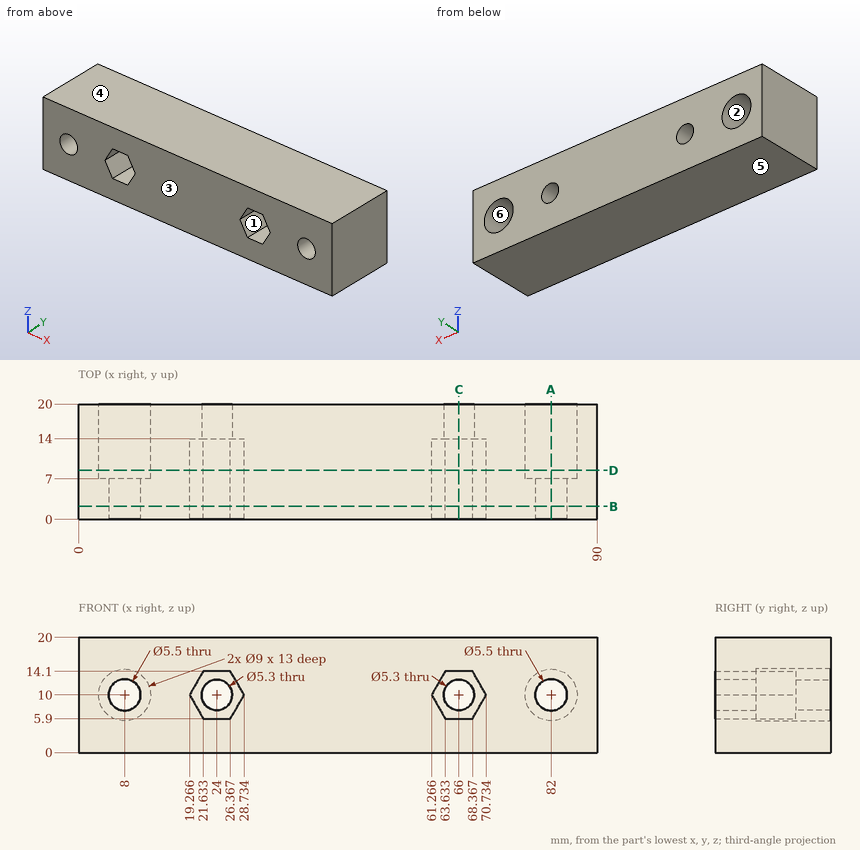
Answer from the drawing. Dimensions are ordinates in mm from the lowest x, y and z of the part. A direction names the side the tool comes from. Coordinates: 2 decimals unless noted, no trailing zeros. Loops run counter-clockwise (first coordinate to the right, second up) from the corner with the lowest first, then second, coordinate; pieces in that order, holes last. Notation, with made-up numbers: (-1.5, 38.25) - (54.5, 38.25) arc R17 ccw to (54.5, 70.25) - close; hole circle Ø1 at (30, 67.25). An arc over 180 degrees is marked (long way). Answer in a Markdown table with one row per item.
1. Straight lines are drawn through the part: line 1 (X direction, y = 10.5, z = 10) (1 decimal); line 2 (X direction, y = 18.4, z = 10); line 3 (X direction, y = 19, z = 13.25). For each, find the intervals that lie inside material, in ascending order.
Conclusion:
| item | result |
|---|---|
| line 1 | x = 0 to 3.5, 12.5 to 19.3, 28.7 to 61.3, 70.7 to 77.5, 86.5 to 90 |
| line 2 | x = 0 to 3.5, 12.5 to 21.35, 26.65 to 63.35, 68.65 to 77.5, 86.5 to 90 |
| line 3 | x = 0 to 4.89, 11.11 to 78.89, 85.11 to 90 |
2. Which of the six approach directions +Z, -Z, +X, -X, +Y, -Y give full straight-line access (tool end or side, diameter ignored) to the marked faces 1, 2 and 3?
Conclusion:
| item | result |
|---|---|
| face 1 | -Y |
| face 2 | +Y |
| face 3 | +Z, -Z, +X, -X, -Y |
3. Given pin 1 (4 mm diameter, centred on x = 26, z = 9.5, fed in from -Y), flat-ended and moving along its own axis, determine where the tip first touches the part or whether it passes through.
Conclusion:
| item | result |
|---|---|
| pin 1 | stops at y = 14 |
4. Find section C-C, the plane x = 66. Write down the section's boundary in (y, z), then the cut area to 3 significant figures.
Conclusion:
| item | result |
|---|---|
| outline | (0, 0) - (20, 0) - (20, 7.35) - (14, 7.35) - (14, 5.9) - (0, 5.9) - close; (0, 14.1) - (14, 14.1) - (14, 12.65) - (20, 12.65) - (20, 20) - (0, 20) - close |
| area | 253 mm² |
5. Determine the mould class of the marked faces 4, 5 and 6 for opening direction Z: +Z half, -Z half, draft (parallel to the pull), parting line (faces both ways), or undercut.
Conclusion:
| item | result |
|---|---|
| face 4 | +Z half |
| face 5 | -Z half |
| face 6 | undercut |
6. Find section D-D, the plane y = 8.5. Write down the section's boundary in (x, z).
Conclusion:
| item | result |
|---|---|
| outline | (0, 0) - (90, 0) - (90, 20) - (0, 20) - close; hole circle Ø9 at (8, 10); hole (19.27, 10) - (21.63, 5.9) - (26.37, 5.9) - (28.73, 10) - (26.37, 14.1) - (21.63, 14.1) - close; hole (61.27, 10) - (63.63, 5.9) - (68.37, 5.9) - (70.73, 10) - (68.37, 14.1) - (63.63, 14.1) - close; hole circle Ø9 at (82, 10) |
7. Find section A-A, the plane x = 82. Write down the section's boundary in (y, z).
Conclusion:
| item | result |
|---|---|
| outline | (0, 0) - (20, 0) - (20, 5.5) - (7, 5.5) - (7, 7.25) - (0, 7.25) - close; (0, 12.75) - (7, 12.75) - (7, 14.5) - (20, 14.5) - (20, 20) - (0, 20) - close |
8. Find section B-B, the plane y = 2.25. Write down the section's boundary in (x, z), then the cut area to 3 significant figures.
Conclusion:
| item | result |
|---|---|
| outline | (0, 0) - (90, 0) - (90, 20) - (0, 20) - close; hole circle Ø5.5 at (8, 10); hole (19.27, 10) - (21.63, 5.9) - (26.37, 5.9) - (28.73, 10) - (26.37, 14.1) - (21.63, 14.1) - close; hole (61.27, 10) - (63.63, 5.9) - (68.37, 5.9) - (70.73, 10) - (68.37, 14.1) - (63.63, 14.1) - close; hole circle Ø5.5 at (82, 10) |
| area | 1,640 mm² |
